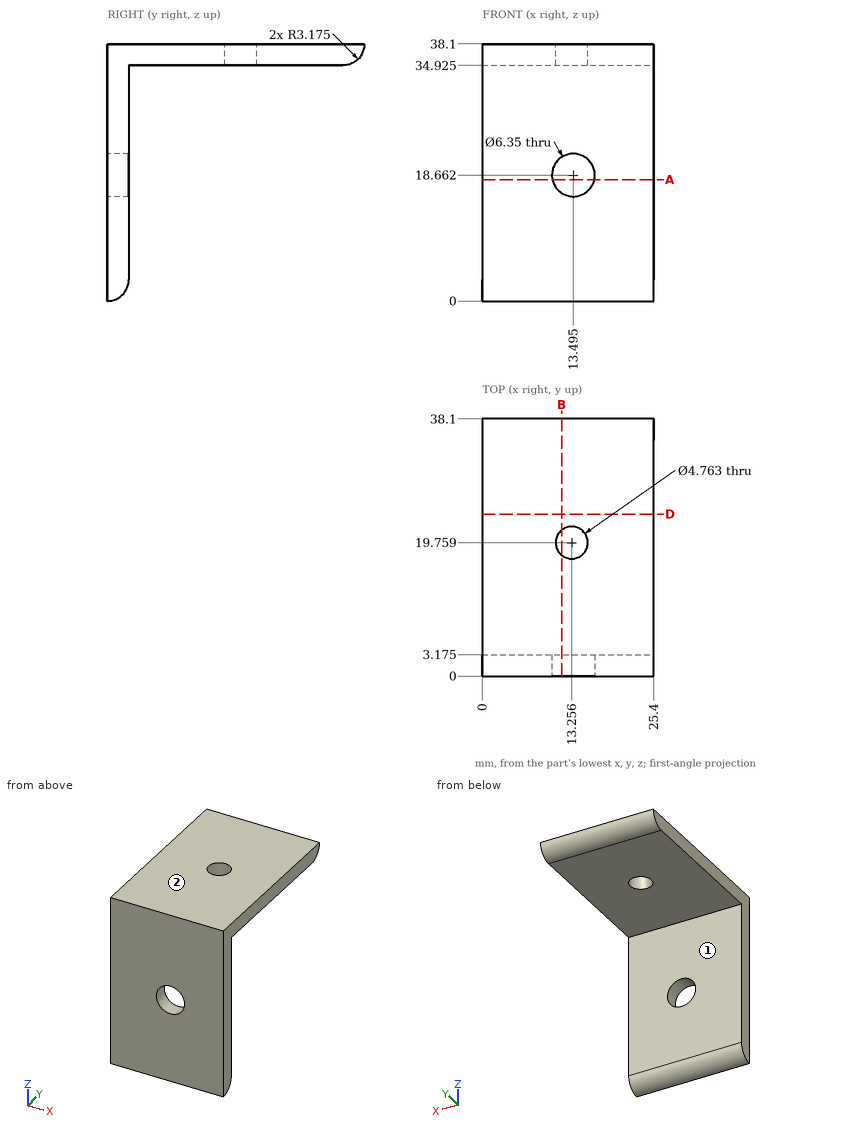
Here's the drawing with two shaded views (mm, measured from the low corner). I have some questions. A direction names the side the tool comes from. Coordinates: 2 decimals unless noted, no trailing zeros. Loops run counter-clockwise (first coordinate to the right, second up) from the corner with the lowest first, then second, coordinate; pieces in that order, holes last. Notation, with made-up numbers: (3.25, 64.25) -> (62.25, 64.25) arc R18 cw to (62.25, 70.25) -> close; hole circle Ø10 at (71, -29.75). An arc over 180 degrees is marked (long way). Put each result on its own line as item: value. Start each with the question number.
Q1. I'm going to push flat-ended pins straight in: P1, Ø10, axis at x = 13.5, z = 18.66, coming from the -Y side; P2, Ø10, axis at x = 7.5, y = 20.5, coming from the -Z side (1 decimal); P3, Ø12.5, axis at x = 13, z = 24, coming from the +Y side (1 decimal). Where does each tip first touch, or does it pass through?
Q2. If I drill on line 1 (Z direction, x = 19.5, y = 13) (1 decimal); line 2 (Y direction, x = 24.25, z = 31) (1 decimal); line 3 (Z direction, x = 15.75, y = 2) (1 decimal), over which ranges is the centre line in solid material (lowest first)? Write a range as [from, to].
Q3. I want a section at D-D (y = 24). Write out the boundary of the cut face in (x, z) (1 decimal).
Q4. I want a section at A-A (z = 18). Write out the boundary of the cut face in (x, y) (1 decimal).
Q5. I want a section at B-B (x = 11.75). Count the separate pieces of the cut face and the enclosed holes in it, plus the area to 3 significant figures.
Q6. For the marked faces 1 and 2, which set-ups out of +Z, -Z, +X, -X, +Y, -Y let a thin tool reach every point of the face, with its end or its side?
Taken from the geometry:
1. P1: stops at y = 0
1. P2: stops at z = 34.9
1. P3: stops at y = 3.2
2. line 1: z = [34.9, 38.1]
2. line 2: y = [0, 3.2]
2. line 3: z = [0.7, 16.4], [20.9, 38.1]
3. outline: (0, 34.9) -> (25.4, 34.9) -> (25.4, 38.1) -> (0, 38.1) -> close
4. outline: (0, 0) -> (10.4, 0) -> (10.4, 3.2) -> (0, 3.2) -> close; (16.6, 0) -> (25.4, 0) -> (25.4, 3.2) -> (16.6, 3.2) -> close
5. separate pieces: 3
5. enclosed holes: 0
5. area: 199 mm2
6. face 1: -Z, +X, -X, +Y
6. face 2: +Z, +X, -X, +Y, -Y
